```python
from build123d import *

# Parameters (mm, degrees)
IZIM1_W                     = 50
IZIM1_H                     = 100
Y_KSEKLIK_EKSTR_ZYON1_DEPTH = 60
IZIM2_R                     = 10
KES_EKSTR_ZYON2_DEPTH       = 35
IZIM3_R                     = 10
KES_EKSTR_ZYON3_DEPTH       = 35
KES_EKSTR_ZYON4_DEPTH       = 40
KES_EKSTR_ZYON5_DEPTH       = 15
IZIM7_R                     = 5
KES_EKSTR_ZYON6_DEPTH       = 8
IZIM8_W                     = 30
IZIM8_H                     = 10
KES_EKSTR_ZYON7_DEPTH       = 101


with BuildPart() as part:
    # Çizim1 → Yükseklik-Ekstrüzyon1 (new body)
    with BuildSketch(Plane.XY):
        with Locations((25, 50)):
            Rectangle(IZIM1_W, IZIM1_H)
    extrude(amount=Y_KSEKLIK_EKSTR_ZYON1_DEPTH)

    # Çizim2 → Kes-Ekstrüzyon2 (cut)
    with BuildSketch(Plane.XY.offset(60)):
        with BuildLine():
            Line((0, 100), (0, 30))
            Line((0, 30), (10, 30))
            ThreePointArc((10, 30), (25, 45), (40, 30))
            Line((40, 30), (50, 30))
            Line((50, 30), (50, 100))
            Line((50, 100), (0, 100))
        make_face()
        with Locations((25, 30)):
            Circle(IZIM2_R)
    extrude(amount=-KES_EKSTR_ZYON2_DEPTH, mode=Mode.SUBTRACT)

    # Çizim3 → Kes-Ekstrüzyon3 (cut)
    with BuildSketch(Plane.XY.offset(25)):
        with Locations((25, 30)):
            Circle(IZIM3_R)
        with BuildLine():
            Line((15, 57), (15, 87))
            ThreePointArc((15, 87), (25, 97), (35, 87))
            Line((35, 87), (35, 57))
            ThreePointArc((35, 57), (25, 47), (15, 57))
        make_face()
    extrude(amount=-KES_EKSTR_ZYON3_DEPTH, mode=Mode.SUBTRACT)

    # Çizim5 → Kes-Ekstrüzyon4 (cut)
    with BuildSketch(Plane.XY.offset(60)):
        with BuildLine():
            Line((35, 10), (15, 10))
            Line((15, 10), (15, 18.819660113))
            ThreePointArc((15, 18.819660113), (11.306936062, 23.876275643), (10, 30))
            Line((10, 30), (0, 30))
            Line((0, 30), (0, 0))
            Line((0, 0), (50, 0))
            Line((50, 0), (50, 30))
            Line((50, 30), (40, 30))
            ThreePointArc((40, 30), (38.693063938, 23.876275643), (35, 18.819660113))
            Line((35, 18.819660113), (35, 10))
        make_face()
    extrude(amount=-KES_EKSTR_ZYON4_DEPTH, mode=Mode.SUBTRACT)

    # Çizim6 → Kes-Ekstrüzyon5 (cut)
    with BuildSketch(Plane.XY.offset(60)):
        with BuildLine():
            Line((15, 18.819660113), (15, 10))
            Line((15, 10), (35, 10))
            Line((35, 10), (35, 18.819660113))
            ThreePointArc((35, 18.819660113), (25, 15), (15, 18.819660113))
        make_face()
    extrude(amount=-KES_EKSTR_ZYON5_DEPTH, mode=Mode.SUBTRACT)

    # Çizim7 → Kes-Ekstrüzyon6 (cut)
    with BuildSketch(Plane.XZ.offset(-10)):
        with Locations((25, 35)):
            Circle(IZIM7_R)
    extrude(amount=-KES_EKSTR_ZYON6_DEPTH, mode=Mode.SUBTRACT)

    # Çizim8 → Kes-Ekstrüzyon7 (cut, through all)
    with BuildSketch(Plane.XZ):
        with Locations((25, 5)):
            Rectangle(IZIM8_W, IZIM8_H)
    extrude(amount=-KES_EKSTR_ZYON7_DEPTH, mode=Mode.SUBTRACT)


solid = part.part
```
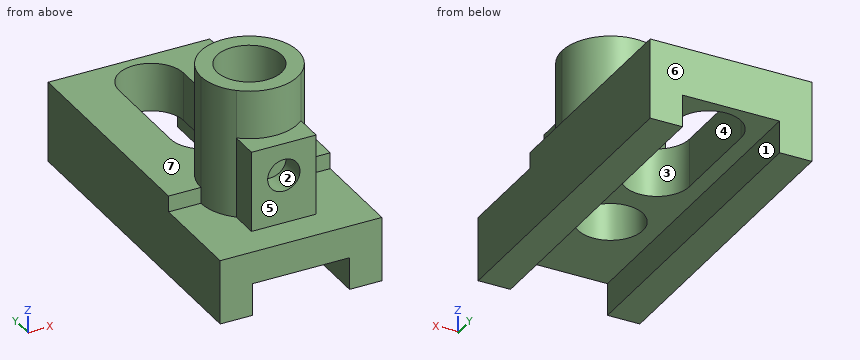
For this review, take the finished solid that the model builds, in its own axes (mm). Face numbers are marked on the shaded views. A direction names the side the tool comes from. Coordinates: 2 decimals unless noted, no trailing zeros. Loops run counter-clockwise (first coordinate to the right, second up) from the corner with the lowest first, then second, coordinate; pieces in that order, holes last.
1. Add section A-A, the plane z = 16. Give the boundary of the cut face in (x, y), then the cut area to 3 significant figures.
2. Mouldability with a two-part tool opening along Y and no side actions: class the marked faces 4, 5, 6 and 7 as +Y half, -Y half, draft (parallel to the pull), parting line (faces both ways), or undercut.
3. Add section C-C, the plane z = 7. Give the boundary of the cut face in (x, y).
4. Add section D-D, the plane y = 24.5. Give the boundary of the cut face in (x, z), then the cut area to 3 significant figures.
5. For line 1 (Z direction, x = 25, y = 16); line 2 (X direction, y = 10.5, z = 5.5); line 3 (Y direction, x = 30.5, z = 13), list the stretches that pass through material, from the lowest coordinate up.
6. Add section B-B, the plane x = 25. Give the boundary of the cut face in (y, z), then the cut area to 3 significant figures.
7. Insertion check: P1, Ø1, axis at x = 14, y = 84.5, coming from the -Z side; P2, Ø8, axis at x = 27, z = 36.5, coming from the -Y side; P3, Ø9, axis at x = 19.5, y = 8, coming from the +Z side; P4, Ø18, axis at x = 25, y = 30, coming from the +Z side. Each pin has a flat end and moves straight along its axis. Give the tip position at first contact, or say it passes through.
8. For the marked faces 1, 2 and 3, list the 3-axis set-ups (+Z, -Z, +X, -X, +Y, -Y) from which the entire face can be reached by the end or side of a thin tool; tool diameter is ignored.
Result:
1. outline: (0, 0) - (50, 0) - (50, 100) - (0, 100) - close; hole circle Ø20 at (25, 30); hole (15, 57) arc R10 ccw to (35, 57) - (35, 87) arc R10 ccw to (15, 87) - close
1. area: 3,770 mm2
2. face 4: undercut
2. face 5: -Y half
2. face 6: +Y half
2. face 7: draft
3. outline: (0, 0) - (10, 0) - (10, 100) - (0, 100) - close; (40, 0) - (50, 0) - (50, 100) - (40, 100) - close
4. outline: (0, 0) - (10, 0) - (10, 10) - (16.65, 10) - (16.65, 60) - (11.04, 60) - (11.04, 20) - (0, 20) - close; (33.35, 10) - (40, 10) - (40, 0) - (50, 0) - (50, 20) - (38.96, 20) - (38.96, 60) - (33.35, 60) - close
4. area: 981 mm2
5. line 1: z = 10 to 30, 40 to 60
5. line 2: x = 0 to 10, 40 to 50
5. line 3: y = 0 to 21.65, 38.35 to 48.65, 95.35 to 100
6. outline: (0, 10) - (20, 10) - (20, 60) - (15, 60) - (15, 45) - (10, 45) - (10, 40) - (18, 40) - (18, 30) - (10, 30) - (10, 20) - (0, 20) - close; (40, 10) - (47, 10) - (47, 25) - (45, 25) - (45, 60) - (40, 60) - close; (97, 10) - (100, 10) - (100, 25) - (97, 25) - close
6. area: 770 mm2
7. P1: stops at z = 10
7. P2: stops at y = 10
7. P3: stops at z = 45
7. P4: passes through
8. face 1: -Z, +Y, -Y
8. face 2: -Y
8. face 3: +Z, -Z
